```python
from build123d import *

# Parameters (mm, degrees)
SKETCH002_W     = 68
SKETCH002_H     = 48
PAD002_DEPTH    = 19
CHAMFER_SIZE2   = 10
CHAMFER_SIZE    = 14
FILLET001_R     = 6.5
THICKNESS_T     = -2
SKETCH004_W     = 18
SKETCH004_H     = 18
POCKET_DEPTH    = 5
POCKET_TAPER    = -12
SKETCH005_W     = 9.5
SKETCH005_H     = 16.4
SKETCH005_W_2   = 11
SKETCH005_H_2   = 12
POCKET001_DEPTH = 5


with BuildPart() as part:
    # Sketch002 → Pad002 (new body)
    with BuildSketch(Plane.XY):
        Rectangle(SKETCH002_W, SKETCH002_H)
    extrude(amount=PAD002_DEPTH)

    # Chamfer
    chamfer_edges = [part.edges().sort_by_distance(p)[0] for p in [
        (34, 0, 19),
    ]]
    chamfer_side = part.faces().sort_by_distance((34, 0, 9.5))[0]
    chamfer(chamfer_edges, length=CHAMFER_SIZE, length2=CHAMFER_SIZE2, reference=chamfer_side)

    # Fillet001
    fillet001_edges = [part.edges().sort_by_distance(p)[0] for p in [
        (29, -24, 12),
        (24, 0, 19),
        (-5, -24, 19),
        (-34, 0, 19),
        (-5, 24, 19),
        (29, 24, 12),
        (34, 0, 5),
        (34, 24, 2.5),
        (34, -24, 2.5),
        (-34, 24, 9.5),
        (-34, -24, 9.5),
    ]]
    fillet(fillet001_edges, radius=FILLET001_R)

    # Thickness
    thickness_openings = [part.faces().sort_by_distance(p)[0] for p in [
        (0, 0, 0),
    ]]
    offset(amount=THICKNESS_T, openings=thickness_openings)

    # Sketch004 (on Face14 of Thickness) → Pocket (cut)
    with BuildSketch(Plane.XY.offset(19)):
        with Locations((15.1, 0)):
            Rectangle(SKETCH004_W, SKETCH004_H)
    extrude(amount=-POCKET_DEPTH, taper=POCKET_TAPER, mode=Mode.SUBTRACT)

    # Sketch005 (on Face7 of Pocket) → Pocket001 (cut)
    with BuildSketch(Plane(origin=(-34, 0, 0), x_dir=(0, -1, 0), z_dir=(-1, 0, 0))):
        with Locations((7.25, 8.2)):
            Rectangle(SKETCH005_W, SKETCH005_H)
        with Locations((-7, 6)):
            Rectangle(SKETCH005_W_2, SKETCH005_H_2)
    extrude(amount=-POCKET001_DEPTH, mode=Mode.SUBTRACT)


solid = part.part
```
The listing builds one solid part. Answer for the finished solid, in the listing's coordinates (mm). A direction names the side the tool comes from. Coordinates: 2 decimals unless noted, no trailing zeros. Loops run counter-clockwise (first coordinate to the right, second up) from the corner with the lowest first, then second, coordinate; pieces in that order, holes last. Notation, with made-up numbers: (28.25, 7.5) -> (53.25, 7.5) arc R28 ccw to (53.25, 34.5) -> close; hole circle Ø3 at (78, 25.5). An arc over 180 degrees is marked (long way). Use one line per item in the form item = value. Start each with the question number.
Item 1: The part is cut by section A-A on y = 11.5. Determine the outline of the cut face in (x, z), then the cut area to 3 significant figures.
Item 2: A tool of negligible diameter and unlimited length cuts with its end or side. For faces 4 (the face through (27.69, -0.24, 10.39)), 5 (the face through (-31, -7, 16.4)), 6 (the face through (27.728, -22.146, 10.418)), from which of +Z, -Z, +X, -X, +Y, -Y can it reach the whole face along a straight path? Write none if from no direction.
Item 3: The part is cut by section B-B on x = -11. Determine the outline of the cut face in (y, z), then the cut area to 3 significant figures.
Item 4: The mould has two halves that part along Y. Classify faces 1 (the face through (0, 24, 6)), 2 (the face through (29, 0, 12)), 3 (the face through (-33, -12, 8)): released by +Y, released by -Y, zero draft, split by the parting line, or undercut.
Item 5: Flat-ended cylindrical pins translate along their axes: pin 1 Ø10 at (x, y) = (21.5, -4.5) entering from -Z; pin 2 Ø2 at (x, z) = (-33.5, 9) entering from +Y; pin 3 Ø6 at (x, y) = (-9, -15.5) entering from -Z. Find the tip coordinate at first contact, or state that the pin passes through.
Item 6: Consider L1, parallel to Y at x = 16, z = 11; L2, parallel to Z at x = -20, y = 6.5; L3, parallel to Y at x = -14.5, z = 13.75. Determine where each line is inside the solid, lowest interval first. Write a range as [from, to].
Answer key:
q1.outline = (-34, 12) -> (-32, 12) -> (-32, 12.5) arc R4.5 cw to (-27.5, 17) -> (20.65, 17) arc R4.5 cw to (24.32, 15.12) -> (31.16, 5.53) arc R4.5 cw to (32, 2.92) -> (32, 0) -> (34, 0) -> (34, 2.92) arc R6.5 ccw to (32.79, 6.7) -> (25.94, 16.28) arc R6.5 ccw to (20.65, 19) -> (-27.5, 19) arc R6.5 ccw to (-34, 12.5) -> close
q1.area = 161 mm2
q2.face_4 = -Z
q2.face_5 = -Z, -X
q2.face_6 = +Z, +X, -Y
q3.outline = (-24, 0) -> (-22, 0) -> (-22, 12.5) arc R4.5 cw to (-17.5, 17) -> (17.5, 17) arc R4.5 cw to (22, 12.5) -> (22, 0) -> (24, 0) -> (24, 12.5) arc R6.5 ccw to (17.5, 19) -> (-17.5, 19) arc R6.5 ccw to (-24, 12.5) -> close
q3.area = 155 mm2
q4.face_1 = released by +Y
q4.face_2 = zero draft
q4.face_3 = undercut
q5.pin_1 = 12.06
q5.pin_2 = 21.65
q5.pin_3 = 16.89
q6.L1 = [-24, -22], [22, 24]
q6.L2 = [17, 19]
q6.L3 = [-23.88, -21.82], [21.82, 23.88]
